Here's how the part is built. I have some questions about the finished solid (model axes, mm). Face numbers are marked on the shaded views. A direction names the side the tool comes from. Round coordinates to 2 decimals unless told otherwise and drop trailing zeros. Order: outer loops, then holes, each group sorted by start corner. A loop starts at its lowest first (then second) coordinate and runs counter-clockwise, first axis right, second up.
```python
from build123d import *

# Parameters (mm, degrees)
SKETCH1_W           = 205
SKETCH1_H           = 165.1
BOSS_EXTRUDE1_DEPTH = 55
CUT_EXTRUDE1_REACH  = 203.964
SKETCH3_W           = 19.95
SKETCH3_H           = 149.1
CUT_EXTRUDE2_DEPTH  = 50
CUT_EXTRUDE3_REACH  = 142.786
SKETCH4_R           = 2.75
FILLET1_R           = 2
SKETCH5_R           = 5.25
CUT_EXTRUDE4_DEPTH  = 10
CUT_EXTRUDE5_REACH  = 144.639
SKETCH6_W           = 80
SKETCH6_H           = 135.1
FILLET2_R           = 20


with BuildPart() as part:
    # Sketch1 → Boss-Extrude1 (new body)
    with BuildSketch(Plane(origin=(0, 0, 0), x_dir=(1, 0, 0), z_dir=(0, 1, 0))):
        Rectangle(SKETCH1_W, SKETCH1_H)
    extrude(amount=BOSS_EXTRUDE1_DEPTH)

    # Sketch2 → Cut-Extrude1 (cut, up to next)
    with BuildSketch(Plane.XY.offset(82.55), mode=Mode.PRIVATE) as cut_extrude1_sk1:
        Polygon((82.55, 55), (102.5, 0), (102.5, 55), align=None)
    cut_extrude1_tool1 = extrude(cut_extrude1_sk1.sketch, amount=-CUT_EXTRUDE1_REACH, mode=Mode.PRIVATE) & part.part
    # Sketch2 → Cut-Extrude1 (cut, up to next)
    with BuildSketch(Plane.XY.offset(82.55), mode=Mode.PRIVATE) as cut_extrude1_sk2:
        Polygon((-82.55, 55), (-102.5, 0), (-102.5, 55), align=None)
    cut_extrude1_tool2 = extrude(cut_extrude1_sk2.sketch, amount=-CUT_EXTRUDE1_REACH, mode=Mode.PRIVATE) & part.part
    add(cut_extrude1_tool1.solids().sort_by_distance((95.85, 36.666667, 82.55))[0], mode=Mode.SUBTRACT)
    add(cut_extrude1_tool2.solids().sort_by_distance((-95.85, 36.666667, 82.55))[0], mode=Mode.SUBTRACT)

    # Sketch3 → Cut-Extrude2 (cut)
    with BuildSketch(Plane(origin=(0, 55, 0), x_dir=(1, 0, 0), z_dir=(0, 1, 0))):
        with Locations((-92.525, 0)):
            Rectangle(SKETCH3_W, SKETCH3_H)
        with Locations((92.525, 0)):
            Rectangle(SKETCH3_W, SKETCH3_H)
    extrude(amount=-CUT_EXTRUDE2_DEPTH, mode=Mode.SUBTRACT)

    # Sketch4 → Cut-Extrude3 (cut, up to next)
    with BuildSketch(Plane(origin=(0, 5, 0), x_dir=(1, 0, 0), z_dir=(0, 1, 0)), mode=Mode.PRIVATE) as cut_extrude3_sk1:
        with Locations(Location((-92.5, 53.71150957, 0), (0, 0, 270))):
            Circle(SKETCH4_R)
    cut_extrude3_tool1 = extrude(cut_extrude3_sk1.sketch, amount=-CUT_EXTRUDE3_REACH, mode=Mode.PRIVATE) & part.part
    # Sketch4 → Cut-Extrude3 (cut, up to next)
    with BuildSketch(Plane(origin=(0, 5, 0), x_dir=(1, 0, 0), z_dir=(0, 1, 0)), mode=Mode.PRIVATE) as cut_extrude3_sk2:
        with Locations(Location((-92.5, 0, 0), (0, 0, 270))):
            Circle(SKETCH4_R)
    cut_extrude3_tool2 = extrude(cut_extrude3_sk2.sketch, amount=-CUT_EXTRUDE3_REACH, mode=Mode.PRIVATE) & part.part
    # Sketch4 → Cut-Extrude3 (cut, up to next)
    with BuildSketch(Plane(origin=(0, 5, 0), x_dir=(1, 0, 0), z_dir=(0, 1, 0)), mode=Mode.PRIVATE) as cut_extrude3_sk3:
        with Locations(Location((-92.5, -53.71150957, 0), (0, 0, 90))):
            Circle(SKETCH4_R)
    cut_extrude3_tool3 = extrude(cut_extrude3_sk3.sketch, amount=-CUT_EXTRUDE3_REACH, mode=Mode.PRIVATE) & part.part
    # Sketch4 → Cut-Extrude3 (cut, up to next)
    with BuildSketch(Plane(origin=(0, 5, 0), x_dir=(1, 0, 0), z_dir=(0, 1, 0)), mode=Mode.PRIVATE) as cut_extrude3_sk4:
        with Locations(Location((92.5, -53.71150957, 0), (0, 0, 270))):
            Circle(SKETCH4_R)
    cut_extrude3_tool4 = extrude(cut_extrude3_sk4.sketch, amount=-CUT_EXTRUDE3_REACH, mode=Mode.PRIVATE) & part.part
    # Sketch4 → Cut-Extrude3 (cut, up to next)
    with BuildSketch(Plane(origin=(0, 5, 0), x_dir=(1, 0, 0), z_dir=(0, 1, 0)), mode=Mode.PRIVATE) as cut_extrude3_sk5:
        with Locations(Location((92.5, 0, 0), (0, 0, 90))):
            Circle(SKETCH4_R)
    cut_extrude3_tool5 = extrude(cut_extrude3_sk5.sketch, amount=-CUT_EXTRUDE3_REACH, mode=Mode.PRIVATE) & part.part
    # Sketch4 → Cut-Extrude3 (cut, up to next)
    with BuildSketch(Plane(origin=(0, 5, 0), x_dir=(1, 0, 0), z_dir=(0, 1, 0)), mode=Mode.PRIVATE) as cut_extrude3_sk6:
        with Locations(Location((92.5, 53.71150957, 0), (0, 0, 90))):
            Circle(SKETCH4_R)
    cut_extrude3_tool6 = extrude(cut_extrude3_sk6.sketch, amount=-CUT_EXTRUDE3_REACH, mode=Mode.PRIVATE) & part.part
    add(cut_extrude3_tool1.solids().sort_by_distance((-92.5, 5, -53.71151))[0], mode=Mode.SUBTRACT)
    add(cut_extrude3_tool2.solids().sort_by_distance((-92.5, 5, 0))[0], mode=Mode.SUBTRACT)
    add(cut_extrude3_tool3.solids().sort_by_distance((-92.5, 5, 53.71151))[0], mode=Mode.SUBTRACT)
    add(cut_extrude3_tool4.solids().sort_by_distance((92.5, 5, 53.71151))[0], mode=Mode.SUBTRACT)
    add(cut_extrude3_tool5.solids().sort_by_distance((92.5, 5, 0))[0], mode=Mode.SUBTRACT)
    add(cut_extrude3_tool6.solids().sort_by_distance((92.5, 5, -53.71151))[0], mode=Mode.SUBTRACT)

    # Fillet1
    fillet1_edges = [part.edges().sort_by_distance(p)[0] for p in [
        (-91.618181818, 5, -74.55),
        (-82.55, 30, 74.55),
        (-91.618181818, 5, 74.55),
        (-82.55, 5, 0),
        (-82.55, 30, -74.55),
        (91.618181818, 5, 74.55),
        (82.55, 30, -74.55),
        (91.618181818, 5, -74.55),
        (82.55, 5, 0),
        (82.55, 30, 74.55),
    ]]
    fillet(fillet1_edges, radius=FILLET1_R)

    # Sketch5 → Cut-Extrude4 (cut)
    with BuildSketch(Plane(origin=(0, 55, 0), x_dir=(1, 0, 0), z_dir=(0, 1, 0))):
        with Locations(Location((63.5, -69.85, 0), (0, 0, 270))):
            Circle(SKETCH5_R)
        with Locations(Location((63.5, 57.15, 0), (0, 0, 270))):
            Circle(SKETCH5_R)
    cut_extrude4 = extrude(amount=-CUT_EXTRUDE4_DEPTH, mode=Mode.SUBTRACT)

    # Mirror1: Cut-Extrude4 across plane
    add(cut_extrude4.mirror(Plane(origin=(0, 0, 0), x_dir=(0, 0, 1), z_dir=(1, 0, 0))), mode=Mode.SUBTRACT)

    # Sketch6 → Cut-Extrude5 (cut, up to next)
    with BuildSketch(Plane(origin=(0, 55, 0), x_dir=(1, 0, 0), z_dir=(0, 1, 0)), mode=Mode.PRIVATE) as cut_extrude5_sk1:
        Rectangle(SKETCH6_W, SKETCH6_H)
    cut_extrude5_tool1 = extrude(cut_extrude5_sk1.sketch, amount=-CUT_EXTRUDE5_REACH, mode=Mode.PRIVATE) & part.part
    add(cut_extrude5_tool1.solids().sort_by_distance((0, 55, 0))[0], mode=Mode.SUBTRACT)

    # Fillet2
    fillet2_edges = [part.edges().sort_by_distance(p)[0] for p in [
        (40, 27.5, -67.55),
        (40, 27.5, 67.55),
        (-40, 27.5, 67.55),
        (-40, 27.5, -67.55),
    ]]
    fillet(fillet2_edges, radius=FILLET2_R)


solid = part.part
```
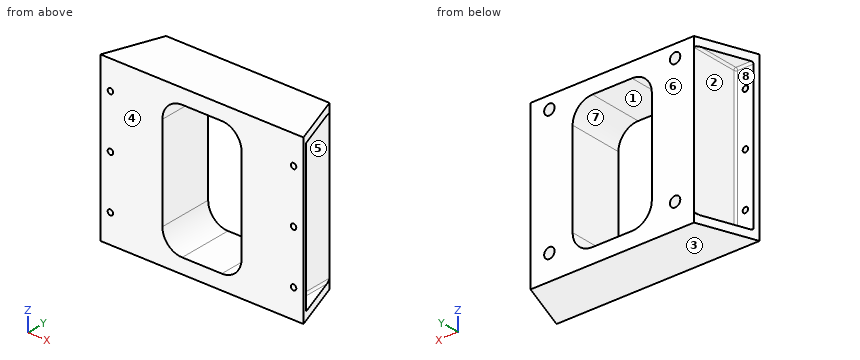
1. If we mould it in two halves opening along X, with no side actions, what happens to the marked faces 1, 2 and 3? For each: released by +X, released by -X, zero draft, split by the parting line, or undercut.
Evaluation:
face 1: undercut
face 2: released by -X
face 3: zero draft
2. I'm going to push flat-ended pins straight in: P1, Ø10, axis at y = 13.5, z = -39.5, coming from the -X side; P2, Ø6.5, axis at x = 92.5, z = 0, coming from the +Y side; P3, Ø8, axis at y = 13.5, z = -56, coming from the +X side. Where does each tip first touch, or does it pass through?
Evaluation:
P1: stops at x = -82.55
P2: stops at y = 5
P3: stops at x = 82.55
3. I need wall thicknesses on probe 1 along Z at (x, y) = (-63, 47); probe 2 along Z at (x, y) = (92, 3); probe 3 along X at (y, z) = (49, 69.85). Which ranges of each line are inside material? Lowest first, please.
Evaluation:
probe 1: z = -82.55 to -62.38, -51.92 to 64.62, 75.08 to 82.55
probe 2: z = -82.55 to -56.42, -51.01 to -2.7, 2.7 to 51.01, 56.42 to 82.55
probe 3: x = -82.55 to -68.75, -58.25 to 58.25, 68.75 to 82.55
4. If we section it at B-B, the plane x = -5.5: Write out the boundary of the cut face in (y, z), and give its area (3 significant figures).
Evaluation:
outline: (0, -82.55) - (55, -82.55) - (55, -67.55) - (0, -67.55) - close; (0, 67.55) - (55, 67.55) - (55, 82.55) - (0, 82.55) - close
area: 1,650 mm2
5. On a 3-axis mill with a long thin cutter (end or side, diameter ignored), from which of +Z, -Z, +X, -X, +Y, -Y can I reach the whole of each face in a straight line? I mean the marked faces 4, 5, 6, 7 and 8. Say none if no direction works.
Evaluation:
face 4: +Z, -Z, +X, -X, -Y
face 5: +X, +Y
face 6: +Z, -Z, +X, -X, +Y
face 7: +Y, -Y
face 8: -X, +Y
6. If we section it at C-C, the plane x = -63.5: Write out the boundary of the cut face in (y, z).
Evaluation:
outline: (0, -82.55) - (55, -82.55) - (55, -62.4) - (45, -62.4) - (45, -51.9) - (55, -51.9) - (55, 64.6) - (45, 64.6) - (45, 75.1) - (55, 75.1) - (55, 82.55) - (0, 82.55) - close
7. If we section it at A-A, the plane z = 5.5: Write out the boundary of the cut face in (x, y), and give its area (3 significant figures).
Evaluation:
outline: (-102.5, 0) - (-40, 0) - (-40, 55) - (-82.55, 55) - (-82.55, 7) arc R2 cw to (-84.55, 5) - (-100.69, 5) - close; (40, 0) - (102.5, 0) - (100.69, 5) - (84.55, 5) arc R2 cw to (82.55, 7) - (82.55, 55) - (40, 55) - close
area: 4,870 mm2
8. If we section it at D-D, the plane y = 35: Write out the boundary of the cut face in (x, z), and give its area (3 significant figures).
Evaluation:
outline: (-89.8, -82.55) - (89.8, -82.55) - (89.8, -74.55) - (84.55, -74.55) arc R2 cw to (82.55, -72.55) - (82.55, 72.55) arc R2 cw to (84.55, 74.55) - (89.8, 74.55) - (89.8, 82.55) - (-89.8, 82.55) - (-89.8, 74.55) - (-84.55, 74.55) arc R2 cw to (-82.55, 72.55) - (-82.55, -72.55) arc R2 cw to (-84.55, -74.55) - (-89.8, -74.55) - close; hole (-40, -47.55) arc R20 ccw to (-20, -67.55) - (20, -67.55) arc R20 ccw to (40, -47.55) - (40, 47.55) arc R20 ccw to (20, 67.55) - (-20, 67.55) arc R20 ccw to (-40, 47.55) - close
area: 17,000 mm2
